Read the model definition and answer for the solid it produces. Units are mm, in the model's axes. A direction names the side the tool comes from. Give positions to 0.01 mm unless a question says otherwise; leave off trailing zeros. Loops run counter-clockwise (first coordinate to the right, second up) from the corner with the lowest first, then second, coordinate; pieces in that order, holes last. Notation, with made-up numbers: (61, 35) - (115, 35) arc R22 ccw to (115, 66) - close; hole circle Ø6 at (45, 45). An arc over 180 degrees is marked (long way). Use a Markdown table: item, result. Add a question column.
Item 1: Which of the six approach directions +Z, -Z, +X, -X, +Y, -Y give full straight-line access (tool end or side, diameter ignored) to faces 1 (the face through (-2.6, 2, 0)), 2 (the face through (1.2, -1, 2)), 3 (the face through (2, -1, -1.85))?
Item 2: For a pull along X with two mould halves and no side action, classify faces 4 (the face through (0, 3.2, 0)), 5 (the face through (2.6, 2, 0)), 6 (the face through (-2.7, -1, 0)), 7 (the face through (-1.2, -1, 2)) as +X half, -X half, draft (parallel to the pull), parting line (faces both ways), or undercut.
Item 3: A cutting plane is placed at B-B (x = -1.35). Determine the outline of the cut face in (y, z).
Item 4: A cutting plane is placed at D-D (z = -0.45). Determine the outline of the cut face in (x, y), plus the area to 3 significant figures.
Item 5: A cutting plane is placed at C-C (y = 1.55). Determine the outline of the cut face in (x, z), plus the area to 3 significant figures.
Item 6: Each of these flat-tipped pins is pushed along its axis until it touches: P1, Ø1.5, axis at x = -0.5, z = 2, coming from the -Y side; P2, Ø1.4, axis at y = 1.5, z = 0, coming from the +X side; P3, Ø0.8, axis at y = 1.5, z = 0, coming from the -X side. Where does it stop, or does it pass through?
Item 7: A cutting plane is placed at A-A (z = -1.45). Determine the outline of the cut face in (x, y).
Item 8: Consider probe 1 along X at (y, z) = (-0.9, 1.3); probe 2 along Z at (x, y) = (-1.2, 0.15); probe 3 along X at (y, z) = (2.5, 0.75). Determine where each line is inside the solid, lowest interval first. Write a range as [from, to].
from build123d import *

# Parameters (mm, degrees)
EXTRUDE_3_DEPTH      = 3.2
EXTRUDE_3_DEPTH_BACK = 1.2
SKETCH_2_W           = 5.4
SKETCH_2_H           = 2.5
EXTRUDE_4_DEPTH      = 1.2
SKETCH_5_W           = 4
SKETCH_5_H           = 1.5
EXTRUDE_7_DEPTH      = 0.5
SKETCH_6_W           = 1.5
SKETCH_6_H           = 1.2
EXTRUDE_8_DEPTH      = 0.6
SKETCH_7_W           = 1.5
SKETCH_7_H           = 1.2
EXTRUDE_9_DEPTH      = 1.5
CHAMFER_2_SIZE       = 0.7


with BuildPart() as part:
    # 草图1 → 凸台-拉伸3 (new, two sides: drawn at the far end of the back side and taken through both)
    with BuildSketch(Plane(origin=(0, 0, 0), x_dir=(1, 0, 0), z_dir=(0, 1, 0)).offset(-EXTRUDE_3_DEPTH_BACK)):
        with BuildLine():
            Line((-2.6, 0.85), (-2.6, -0.85))
            ThreePointArc((-2.6, -0.85), (-2.482842712, -1.132842712), (-2.2, -1.25))
            Line((-2.2, -1.25), (2.2, -1.25))
            ThreePointArc((2.2, -1.25), (2.482842712, -1.132842712), (2.6, -0.85))
            Line((2.6, -0.85), (2.6, 0.85))
            ThreePointArc((2.6, 0.85), (2.482842712, 1.132842712), (2.2, 1.25))
            Line((2.2, 1.25), (-2.2, 1.25))
            ThreePointArc((-2.2, 1.25), (-2.482842712, 1.132842712), (-2.6, 0.85))
        make_face()
    extrude(amount=EXTRUDE_3_DEPTH + EXTRUDE_3_DEPTH_BACK)

    # 草图2 → 凸台-拉伸4 (add)
    with BuildSketch(Plane(origin=(0, 0, 0), x_dir=(1, 0, 0), z_dir=(0, 1, 0))):
        Rectangle(SKETCH_2_W, SKETCH_2_H)
    extrude(amount=-EXTRUDE_4_DEPTH)

    # 草图5 → 凸台-拉伸7 (add)
    with BuildSketch(Plane(origin=(0, -1.2, 0), x_dir=(-1, 0, 0), z_dir=(0, -1, 0))):
        with Locations((0, 0.15)):
            Rectangle(SKETCH_5_W, SKETCH_5_H)
    extrude(amount=EXTRUDE_7_DEPTH)

    # 草图6 → 凸台-拉伸8 (add)
    with BuildSketch(Plane(origin=(0, 0, -1.25), x_dir=(-1, 0, 0), z_dir=(0, 0, -1))):
        with Locations((1.95, -0.6)):
            Rectangle(SKETCH_6_W, SKETCH_6_H)
        with Locations((-1.95, -0.6)):
            Rectangle(SKETCH_6_W, SKETCH_6_H)
    extrude(amount=EXTRUDE_8_DEPTH)

    # 草图7 → 凸台-拉伸9 (add)
    with BuildSketch(Plane.XY.offset(1.25)):
        with Locations((1.95, -0.6)):
            Rectangle(SKETCH_7_W, SKETCH_7_H)
        with Locations((-1.95, -0.6)):
            Rectangle(SKETCH_7_W, SKETCH_7_H)
    extrude(amount=EXTRUDE_9_DEPTH)

    # 倒角2
    chamfer_2_edges = [part.edges().sort_by_distance(p)[0] for p in [
        (1.95, 0, 2.75),
        (-1.95, 0, 2.75),
    ]]
    chamfer(chamfer_2_edges, length=CHAMFER_2_SIZE)


solid = part.part
Geometry says:
| question | item | result |
|---|---|---|
| 1 | face 1 | +Z, -Z, -X, +Y |
| 1 | face 2 | +Z, +Y, -Y |
| 1 | face 3 | -Z, +X, -X, +Y, -Y |
| 2 | face 4 | draft |
| 2 | face 5 | +X half |
| 2 | face 6 | -X half |
| 2 | face 7 | undercut |
| 3 | outline | (-1.7, -0.9) - (-1.2, -0.9) - (-1.2, -1.85) - (0, -1.85) - (0, -1.25) - (3.2, -1.25) - (3.2, 1.25) - (0, 1.25) - (0, 2.05) - (-0.7, 2.75) - (-1.2, 2.75) - (-1.2, 0.6) - (-1.7, 0.6) - close |
| 4 | outline | (-2.7, -1.2) - (-2, -1.2) - (-2, -1.7) - (2, -1.7) - (2, -1.2) - (2.7, -1.2) - (2.7, 0) - (2.6, 0) - (2.6, 3.2) - (-2.6, 3.2) - (-2.6, 0) - (-2.7, 0) - close |
| 4 | area | 25.1 mm² |
| 5 | outline | (-2.6, -0.85) arc R0.4 ccw to (-2.2, -1.25) - (2.2, -1.25) arc R0.4 ccw to (2.6, -0.85) - (2.6, 0.85) arc R0.4 ccw to (2.2, 1.25) - (-2.2, 1.25) arc R0.4 ccw to (-2.6, 0.85) - close |
| 5 | area | 12.9 mm² |
| 6 | P1 | y = -1.2 |
| 6 | P2 | x = 2.6 |
| 6 | P3 | x = -2.6 |
| 7 | outline | (-2.7, -1.2) - (-1.2, -1.2) - (-1.2, 0) - (-2.7, 0) - close; (1.2, -1.2) - (2.7, -1.2) - (2.7, 0) - (1.2, 0) - close |
| 8 | probe 1 | [-2.7, -1.2], [1.2, 2.7] |
| 8 | probe 2 | [-1.25, 1.25] |
| 8 | probe 3 | [-2.6, 2.6] |
